Autodesk Inventor part; units mm, degrees
ref_plane "Plan de construction1" through (5, 0, 0) normal (-1, 0, 0) x (0, 0, 1)
ref_plane "YZ Plane" through (0, 0, 0) normal (1, 0, 0) x (0, 1, 0)
ref_plane "XZ Plane" through (0, 0, 0) normal (0, 1, 0) x (-1, 0, 0)
sketch "Esquisse1" plane through (0, 0, 0) normal (1, 0, 0) x (0, 1, 0)
  circle A0 centre (0, 0) radius 16
  line L0 (-16, 0) -> (59, 0)
  line L1 (59, 0) -> (51, 0)
  circle A1 centre (51, 0) radius 5
  circle A2 centre (51, 0) radius 8
  line L2 (0, 16) -> (51, 8)
  line L3 (51, -8) -> (0, -16)
  circle A3 centre (0, 0) radius 11
  line L4 (34.396, -10.6045) -> (34.396, 10.6045)
  dimension "d0" = 32
  dimension "d1" = 75
  dimension "d2" = 8
  dimension "d3" = 10
  dimension "d4" = 16
  dimension "d5" = 22
extrude "Extrusion1" add sketch "Esquisse1" along normal blind 10 contours L2 A0 L0 A3 | L0 A3 A0 L3 | L2 L4 L0 A0 | L0 L4 L3 A0
sketch "Esquisse2" plane through (0, 0, 0) normal (-1, 0, 0) x (0, 0, 1)
  circle A0 centre (0, 0) radius 11
  circle A1 centre (0, 0) radius 4.25
  dimension "d8" = 8.5
extrude "Extrusion2" add sketch "Esquisse2" along normal blind 10
sketch "Esquisse3" plane through (-10, 0, 0) normal (-1, 0, 0) x (0, 0, 1)
  line L0 (0, 0) -> (-10, 0)
  circle A0 centre (0, 0) radius 11
  line L1 (0, 0) -> (0, 10)
  circle A1 centre (0, 0) radius 4.25
  line L2 (0, 0) -> (10, 0)
  line L3 (0, 0) -> (0, -10)
  line L4 (0, 10) -> (-10, 0)
  line L5 (0, 10) -> (10, 0)
  line L6 (10, 0) -> (0, -10)
  line L7 (-10, 0) -> (0, -10)
  circle A2 centre (0, 0) radius 4.25
  dimension "d12" = 10
  dimension "d13" = 10
  dimension "d14" = 10
  dimension "d15" = 10
  dimension "d16" = 8.5
extrude "Extrusion3" add sketch "Esquisse3" along normal blind 5 contours A1 L3 L7 L0 | L0 L4 L1 A1 | L1 L5 L2 A1 | L2 L6 L3 A1
sketch "Esquisse4" plane through (0, 0, 0) normal (-1, 0, 0) x (0, 0, 1)
  circle A0 centre (0, 0) radius 13.75
  circle A1 centre (0, 0) radius 11
  dimension "d19" = 27.5
extrude "Extrusion4" add sketch "Esquisse4" along normal up to surface (10 mm away)
ref_plane "Plan de construction1" through (5, 0, 0) normal (-1, 0, 0) x (0, 0, 1)
sketch "Esquisse7" plane through (5, 0, 0) normal (-1, 0, 0) x (0, 0, 1)
  point P0 (0, 0)
sketch "Esquisse8" plane through (5, 0, 0) normal (-1, 0, 0) x (0, 0, 1)
  circle A0 centre (0, 51) radius 5
  circle A1 centre (0, 51) radius 4.25
  line L0 (-16, 0) -> (-10.6045, 34.396)
  line L1 (10.6045, 34.396) -> (16, 0)
  arc A2 (8, 51) -> (-8, 51) centre (0, 51) ccw
  line L2 (-10.6045, 34.396) -> (10.6045, 34.396)
  line L3 (-10.6045, 34.396) -> (-8, 51)
  line L4 (8, 51) -> (10.6045, 34.396)
  line L5 (10.6045, 34.396) -> (-10.6045, 34.396)
  point P0 (0, 0)
extrude "Extrusion6" add sketch "Esquisse8" along normal mid plane 6.2 contours A0 | L4 L2 L3 A2
fillet "Congé1" radius 10 4 edges at (8.1, 34.396, 0) (1.9, 34.396, 0) (10, 34.396, 0) (0, 34.396, 0)
sketch "Esquisse10" plane through (0, 0, 0) normal (-1, 0, 0) x (0, 0, 1)
  line L0 (-11.0193, 31.7521) -> (11.0193, 31.7521)
  line L1 (-11.0193, 31.7521) -> (11.0193, 31.7521)
  arc A0 (8, 51) -> (-8, 51) centre (0, 51) ccw
  line L2 (-8, 51) -> (-8, 31.7521)
  line L3 (9.6847, 40.2603) -> (8, 51)
  line L4 (8, 51) -> (8, 31.7521)
  arc A1 (8, 51) -> (-8, 51) centre (0, 51) ccw
  line L5 (-11.0193, 31.7521) -> (-8, 51)
  line L6 (8, 51) -> (11.0193, 31.7521)
  point P0 (0, 0)
extrude "Extrusion8" cut sketch "Esquisse10" against normal blind 10 contours L5 L2 L0 | L4 L3 L6 L0
fillet "Congé2" radius 5 2 edges at (5, 31.7521, -8) (5, 31.7521, -11.0193)
fillet "Congé3" radius 5 2 edges at (5, 31.7521, 11.0193) (5, 31.7521, 8)
sketch "Esquisse11" plane through (0, 0, 0) normal (1, 0, 0) x (0, 0, -1)
  circle A0 centre (0, 0) radius 11
  circle A1 centre (0, 0) radius 7.5
  dimension "d45" = 15
extrude "Extrusion9" add sketch "Esquisse11" along normal blind 3
sketch "Esquisse13" plane through (1.9, 0, 0) normal (-1, 0, 0) x (0, 0, 1)
  circle A0 centre (0, 51) radius 4.25
  circle A1 centre (0, 51) radius 2.75
  point P0 (0, 0)
  dimension "d51" = 5.5
extrude "Extrusion11" add sketch "Esquisse13" against normal up to surface (6.2 mm away)
properties part number "bièlle côté"
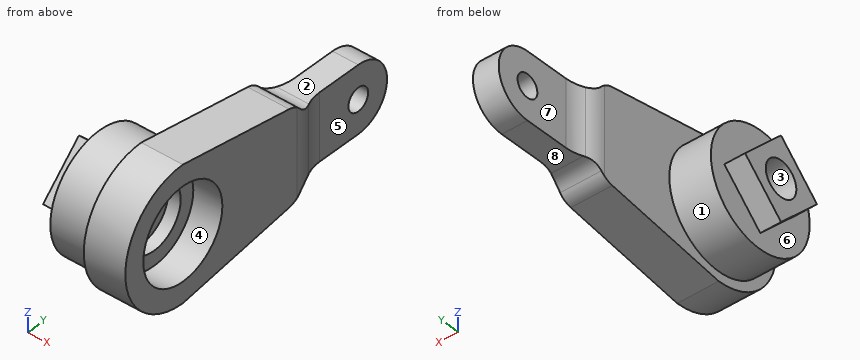
Check sheet for the modelled part. Datum: model origin and axes. Units: mm. Face numbers are marked on the shaded views. A direction names the side the tool comes from. Give positions to 0.01 mm unless a question says otherwise; leave off trailing zeros. Loops run counter-clockwise (first coordinate to the right, second up) from the corner with the lowest first, then second, coordinate; pieces in that order, holes last. Notation, with made-up numbers: M 72,86.25 L 76,86.25 A4 ccw 76,93.25 Z; hole C 31,-35 d2. An arc over 180 degrees is marked long. Use a Markdown table: item, result. Add a question column.
Q1. Sectioned sample at C-C, the plane z = 6.5. Record the cut outline in (x, y), then the cut area to 3 significant figures.
Q2. Sectioned sample at B-B, the plane z = 1.5. Give the number of separate pieces and of enclosed holes in the cut face, then the cut area to 3 significant figures.
Q3. Sectioned sample at D-D, the plane x = -3.75. Record the cut outline in (y, z), then the cut area to 3 significant figures.
Q4. Mould release check, pull along Z, two halves, no side actions. Record for the marked faces 1, 2, 3 and 4: pulls with the +Z half, pulls with the -Z half, needs draft (parallel to the pull), parting line crosses it, or undercut.
Q5. Sectioned sample at A-A, the plane x = 5.5. Record the cut outline in (y, z), then the cut area to 3 significant figures.
Q6. Tool access check on the marked faces 5, 6, 7 and 8. Record the directions out of +Z, -Z, +X, -X, +Y, -Y that give a thin tool (end or side, any length) a straight path to the whole face; none if there is none.
Q7. Scan lines: line 1 along Y through (x, z) = (4.75, 0); line 2 along Z through (x, y) = (6.5, 0); line 3 along Y through (x, z) = (-4.25, -3). Record each from-to range of solid material in increasing order. Write a range as [from, to].
Q8. Go/stop test with flat-tipped pins: pin 1 (9 mm diameter, centred on y = 0, z = 0, fed in from +X); pin 2 (4 mm diameter, centred on x = 4.5, y = 40, fed in from +Z); pin 3 (9 mm diameter, centred on y = 51, z = 0, fed in from -X). Record where each tip stops, or that it passes through.
Verdict:
| question | item | result |
|---|---|---|
| 1 | outline | M -15,-3.5 L -10,-3.5 L -10,-12.12 L 0,-12.12 L 0,-14.62 L 10,-14.62 L 10,-8.87 L 3,-8.87 L 3,-3.74 L 0,-3.74 L 0,3.74 L 3,3.74 L 3,8.87 L 10,8.87 L 10,31.75 A10 ccw 9.05,36.01 A10 cw 8.1,40.26 L 8.1,55.66 L 1.9,55.66 L 1.9,40.26 A10 cw 0.95,36.01 A10 ccw 0,31.75 L 0,12.12 L -10,12.12 L -10,3.5 L -15,3.5 Z |
| 1 | area | 759 mm^2 |
| 2 | separate pieces | 3 |
| 2 | enclosed holes | 0 |
| 2 | area | 675 mm^2 |
| 3 | outline | C 0,0 d27.5; hole C 0,0 d8.5 |
| 3 | area | 537 mm^2 |
| 4 | face 1 | parting line crosses it |
| 4 | face 2 | pulls with the +Z half |
| 4 | face 3 | undercut |
| 4 | face 4 | undercut |
| 5 | outline | M 0,-16 L 29.59,-11.36 A5 ccw 32.58,-9.71 A5 cw 36.34,-8 L 51,-8 A8 ccw 51,8 L 36.34,8 A5 cw 32.58,9.71 A5 ccw 29.59,11.36 L 0,16 A16 ccw Z; hole C 0,0 d22; hole C 51,0 d5.5 |
| 5 | area | 1,270 mm^2 |
| 6 | face 5 | +Z, -Z, +X, +Y |
| 6 | face 6 | -X |
| 6 | face 7 | +Z, -Z, -X, +Y |
| 6 | face 8 | -Z, +X, -X, +Y |
| 7 | line 1 | [-16, -11], [11, 48.25], [53.75, 59] |
| 7 | line 2 | [-16, -11], [11, 16] |
| 7 | line 3 | [-13.42, -3.01], [3.01, 13.42] |
| 8 | pin 1 | x = 0 |
| 8 | pin 2 | z = 8 |
| 8 | pin 3 | x = 1.9 |
